Check sheet for the modelled part. Datum: model origin and axes. Units: mm. Face numbers are marked on the shaded views. A direction names the side the tool comes from. Round coordinates to 2 decimals unless told otherwise and drop trailing zeros. Write each loop counter-clockwise with the first axis right and the second up, starting at its lowest first coordinate (ties: lowest second). Pieces come first, ordered by that corner, then holes. Notation, with made-up numbers: (-21, 36.5) - (-1, 36.5) arc R17 cw to (-1, 49.5) - close; hole circle Ø3 at (42.25, 75). An arc over 180 degrees is marked (long way). Answer as a JSON object with one key per item and string values. Group by question number.
Item 1: Release check for a two-part mould opening along Y. For the marked faces 6, 7 and 8 record: pulls with the +Y half, pulls with the -Y half, needs draft (parallel to the pull), parting line crosses it, or undercut.
Item 2: Thickness scan on line 1 (X direction, y = -3.25, z = 0.25); line 2 (Z direction, x = -25, y = 6.55); line 3 (Z direction, x = -25, y = -6.25). Record the ranges inside material, lowest first.
Item 3: Gauge pin test, flat ends, axial feed: P1, Ø8, axis at y = 4.5, z = -5, coming from the -X side; P2, Ø10.5, axis at x = -22, z = 2.5, coming from the +Y side; P3, Ø10, axis at x = -25, z = 0, coming from the +Y side; P4, Ø1, axis at x = 7, y = -4.5, coming from the -Z side. Record the tip position at first contact, or that the pin passes through.
Item 4: Sectioned sample at B-B on x = -25. Count the separate pieces of the cut face and the enclosed holes in it, plus the area to 3 significant figures.
Item 5: Sectioned sample at A-A on y = 7.25. Record the boundary of the cut face in (x, z).
Item 6: Sectioned sample at C-C on y = -1.75. Record the boundary of the cut face in (x, z).
Item 7: Set-up check for the marked faces 1, 2, 3, 4 and 5: record each of +Z, -Z, +X, -X, +Y, -Y from which the full face is reachable in a straight line by a thin tool's end or side.
```python
from build123d import *

# Parameters (mm, degrees)
F1_DEPTH  = 10
F3_R      = 3.25
F4_DEPTH  = 20.001
F2_R      = 4.25
F5_DEPTH  = 9
F6_R      = 6.55
F6_R_2    = 4.25
F7_DEPTH  = 5.5
F8_R      = 11
F9_DEPTH  = 5
F11_DEPTH = 5
F12_R     = 2
F14_W     = 6
F14_H     = 30
F15_DEPTH = 40
F16_R     = 2.5
F17_SIZE  = 0.5


with BuildPart() as f1:
    # F0 (on Front) → F1 (new body, symmetric)
    with BuildSketch(Plane.XZ):
        with BuildLine():
            ThreePointArc((20.4918032787, 10.0337511591), (0, 5.641710973), (-20.4918032787, 10.0337511591))
            ThreePointArc((-20.4918032787, 10.0337511591), (-36, 0), (-20.4918032787, -10.0337511591))
            ThreePointArc((-20.4918032787, -10.0337511591), (0, -5.641710973), (20.4918032787, -10.0337511591))
            ThreePointArc((20.4918032787, -10.0337511591), (36, 0), (20.4918032787, 10.0337511591))
        make_face()
    extrude(amount=F1_DEPTH, both=True)

    # F3 (on face) → F4 (cut, through all)
    with BuildSketch(Plane(origin=(0, 10, 0), x_dir=(-1, 0, 0), z_dir=(0, 1, 0))):
        with Locations((-25, 0)):
            Circle(F3_R)
        with Locations((25, 0)):
            Circle(F3_R)
    extrude(amount=-F4_DEPTH, mode=Mode.SUBTRACT)

    # F2 (on face) → F5 (cut)
    with BuildSketch(Plane(origin=(0, 10, 0), x_dir=(-1, 0, 0), z_dir=(0, 1, 0))):
        with Locations((25, 0)):
            Circle(F2_R)
    extrude(amount=-F5_DEPTH, mode=Mode.SUBTRACT)

    # F6 (on face) → F7 (cut)
    with BuildSketch(Plane(origin=(0, 10, 0), x_dir=(-1, 0, 0), z_dir=(0, 1, 0))):
        with Locations((25, 0)):
            Circle(F6_R)
        with Locations((25, 0)):
            Circle(F6_R_2, mode=Mode.SUBTRACT)
    extrude(amount=-F7_DEPTH, mode=Mode.SUBTRACT)

    # F8 (on face) → F9 (cut)
    with BuildSketch(Plane.XZ.offset(10)):
        with BuildLine():
            ThreePointArc((5.6538687387, -7.9576025909), (-2.1053254823, -4.6082797346), (-9.1895908953, 0))
            ThreePointArc((-9.1895908953, 0), (-2.1053254823, 4.6082797346), (5.6538687387, 7.9576025909))
            Line((5.6538687387, 7.9576025909), (-41.2745177746, 16.0983856767))
            Line((-41.2745177746, 16.0983856767), (-41.2745177746, 0))
            Line((-41.2745177746, 0), (-41.2745177746, -16.0983856767))
            Line((-41.2745177746, -16.0983856767), (5.6538687387, -7.9576025909))
        make_face()
        with Locations((-25, 0)):
            Circle(F8_R, mode=Mode.SUBTRACT)
    extrude(amount=-F9_DEPTH, mode=Mode.SUBTRACT)

    # F10 (on face) → F11 (cut)
    with BuildSketch(Plane(origin=(0, 10, 0), x_dir=(-1, 0, 0), z_dir=(0, 1, 0))):
        with BuildLine():
            Line((-5.6538687387, -7.9576025909), (41.2745177746, -16.0983856767))
            Line((41.2745177746, -16.0983856767), (41.2745177746, 0))
            Line((41.2745177746, 0), (41.2745177746, 16.0983856767))
            Line((41.2745177746, 16.0983856767), (-5.6538687387, 7.9576025909))
            ThreePointArc((-5.6538687387, 7.9576025909), (-2.7576543334, 6.8880347996), (0.0670265411, 5.6417558986))
            ThreePointArc((0.0670265411, 5.6417558986), (10.5113641589, 6.7590839617), (20.4918032787, 10.0337511591))
            ThreePointArc((20.4918032787, 10.0337511591), (30.9753592388, 9.235533659), (36, 0))
            ThreePointArc((36, 0), (30.9753592388, -9.235533659), (20.4918032787, -10.0337511591))
            ThreePointArc((20.4918032787, -10.0337511591), (10.5113641589, -6.7590839617), (0.0670265411, -5.6417558986))
            ThreePointArc((0.0670265411, -5.6417558986), (-2.7576543334, -6.8880347996), (-5.6538687387, -7.9576025909))
        make_face()
        with BuildLine():
            ThreePointArc((9.1895908953, 0), (4.7800323728, -3.0662109323), (0.0670265411, -5.6417558986))
            ThreePointArc((0.0670265411, -5.6417558986), (10.5113641589, -6.7590839617), (20.4918032787, -10.0337511591))
            ThreePointArc((20.4918032787, -10.0337511591), (14, 0), (20.4918032787, 10.0337511591))
            ThreePointArc((20.4918032787, 10.0337511591), (10.5113641589, 6.7590839617), (0.0670265411, 5.6417558986))
            ThreePointArc((0.0670265411, 5.6417558986), (4.7800323728, 3.0662109323), (9.1895908953, 0))
        make_face()
    extrude(amount=-F11_DEPTH, mode=Mode.SUBTRACT)

    # F12
    f12_edges = [f1.edges().sort_by_distance(p)[0] for p in [
        (-36, -10, 0),
        (-4.780032, -10, -3.066211),
        (-4.780032, -10, 3.066211),
        (10.445826, -10, 6.745037),
        (10.445826, 10, -6.745037),
        (-4.780032, 10, -3.066211),
        (-4.780032, 10, 3.066211),
        (-29.508197, 10, -10.033751),
    ]]
    fillet(f12_edges, radius=F12_R)

    # F14 (on offset) → F15 (cut)
    with BuildSketch(Plane.YZ.offset(-36)):
        Rectangle(F14_W, F14_H)
    extrude(amount=F15_DEPTH, mode=Mode.SUBTRACT)

    # F16
    f16_edges = [f1.edges().sort_by_distance(p)[0] for p in [
        (4, 3, 0),
        (4, -3, 0),
    ]]
    fillet(f16_edges, radius=F16_R)

    # F17
    f17_edges = [f1.edges().sort_by_distance(p)[0] for p in [
        (-21.75, -10, 0),
        (28.25, -10, 0),
        (28.25, 10, 0),
    ]]
    chamfer(f17_edges, length=F17_SIZE)


solid = f1.part
```
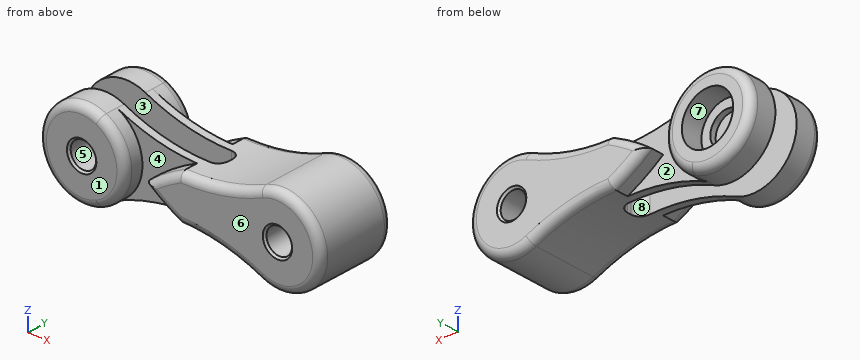
Completed:
{
 "1": {"face 6": "pulls with the -Y half", "face 7": "needs draft", "face 8": "undercut"},
 "2": {"line 1": "-36 to -28.24, -21.76 to 21.76, 28.24 to 36", "line 2": "-11 to -6.55, 6.55 to 11", "line 3": "-11 to -3.25, 3.25 to 11"},
 "3": {"P1": "x = -35.95", "P2": "y = 10", "P3": "y = 4.5", "P4": "z = -6.21"},
 "4": {"separate pieces": "4", "enclosed holes": "0", "area": "174 mm²"},
 "5": {"outline": "circle Ø22 at (-25, 0); (-9.19, 0) arc R50 ccw to (-0.07, -5.64) arc R50 cw to (20.49, -10.03) arc R11 ccw (long way) to (20.49, 10.03) arc R50 cw to (-0.07, 5.64) arc R50 ccw to start; hole circle Ø13.1 at (-25, 0); hole circle Ø6.5 at (25, 0)"},
 "6": {"outline": "(3.67, -5.78) arc R50 cw to (20.49, -10.03) arc R11 ccw (long way) to (20.49, 10.03) arc R50 cw to (3.67, 5.78) - close; hole circle Ø6.5 at (25, 0)"},
 "7": {"face 1": "+Z, -Z, +X, -X, -Y", "face 2": "+Y", "face 3": "+Z, -Z, -X", "face 4": "-Y", "face 5": "+Y, -Y"}
}
